The listing builds one solid part. Answer for the finished solid, in the listing's coordinates (mm). A direction names the side the tool comes from. Give positions to 0.01 mm unless a question says otherwise; leave off trailing zeros. Loops run counter-clockwise (first coordinate to the right, second up) from the corner with the lowest first, then second, coordinate; pieces in that order, holes last. Notation, with made-up numbers: M -39.5,83 L -21.5,83 A24 ccw -21.5,102 Z; hole C -26,-23.5 d9. An arc over 180 degrees is marked long. Return JSON: item names as keys, results as strings.
from build123d import *

# Parameters (mm, degrees)
SCHIZZO16_W                   = 10
SCHIZZO16_H                   = 180
SCHIZZO17_R                   = 20
ESTRUSIONE_ESTRUSIONE10_DEPTH = 12.75569081
SCHIZZO18_R                   = 8.5
ESTRUSIONE_ESTRUSIONE11_DEPTH = 32
SCHIZZO19_R                   = 6
ESTRUSIONE_ESTRUSIONE12_DEPTH = 44
SCHIZZO20_R                   = 5
ESTRUSIONE_ESTRUSIONE13_DEPTH = 10
SCHIZZO21_R                   = 4
ESTRUSIONE_ESTRUSIONE14_DEPTH = 12
SCHIZZO22_R                   = 20
ESTRUSIONE_ESTRUSIONE15_DEPTH = 11.80548778
SCHIZZO23_R                   = 7.4
ESTRUSIONE_ESTRUSIONE16_DEPTH = 61.8
SCHIZZO24_R                   = 5
ESTRUSIONE_ESTRUSIONE17_DEPTH = 10
RACCORDO1_R                   = 100


with BuildPart() as part:
    # Sweep1: sweep along a path in Schizzo15
    with BuildLine(Plane(origin=(0, 0, 0), x_dir=(1, 0, 0), z_dir=(0, 1, 0))) as sweep1_path:
        Line((-350, 35.20194684), (-190, 35.20194684))
        Line((-190, 35.20194684), (-80, 0))
        Line((-80, 0), (80, 0))
    # Schizzo16 → Sweep1 (sweep)
    with BuildSketch(Plane(origin=(0, 0, 0), x_dir=(0, 0, -1), z_dir=(1, 0, 0))):
        Rectangle(SCHIZZO16_W, SCHIZZO16_H)
    sweep(path=sweep1_path.line, transition=Transition.RIGHT)

    # Schizzo17 → Estrusione-Estrusione10 (add)
    with BuildSketch(Plane.XY.offset(5)):
        Circle(SCHIZZO17_R)
    extrude(amount=ESTRUSIONE_ESTRUSIONE10_DEPTH)

    # Schizzo18 → Estrusione-Estrusione11 (add)
    with BuildSketch(Plane.XY.offset(17.75569081)):
        Circle(SCHIZZO18_R)
    extrude(amount=ESTRUSIONE_ESTRUSIONE11_DEPTH)

    # Schizzo19 → Estrusione-Estrusione12 (add)
    with BuildSketch(Plane.XY.offset(49.75569081)):
        Circle(SCHIZZO19_R)
    extrude(amount=ESTRUSIONE_ESTRUSIONE12_DEPTH)

    # Schizzo20 → Estrusione-Estrusione13 (add)
    with BuildSketch(Plane.XY.offset(93.75569081)):
        Circle(SCHIZZO20_R)
    extrude(amount=ESTRUSIONE_ESTRUSIONE13_DEPTH)

    # Schizzo21 → Estrusione-Estrusione14 (add)
    with BuildSketch(Plane.XY.offset(103.75569081)):
        Circle(SCHIZZO21_R)
    extrude(amount=ESTRUSIONE_ESTRUSIONE14_DEPTH)

    # Schizzo22 → Estrusione-Estrusione15 (add)
    with BuildSketch(Plane.XY.offset(-30.20194684)):
        with Locations((-270, 0)):
            Circle(SCHIZZO22_R)
    extrude(amount=ESTRUSIONE_ESTRUSIONE15_DEPTH)

    # Schizzo23 → Estrusione-Estrusione16 (add)
    with BuildSketch(Plane.XY.offset(-18.39645906)):
        with Locations((-270, 0)):
            Circle(SCHIZZO23_R)
    extrude(amount=ESTRUSIONE_ESTRUSIONE16_DEPTH)

    # Schizzo24 → Estrusione-Estrusione17 (add)
    with BuildSketch(Plane.XY.offset(43.40354094)):
        with Locations((-270, 0)):
            Circle(SCHIZZO24_R)
    extrude(amount=ESTRUSIONE_ESTRUSIONE17_DEPTH)

    # Raccordo1
    raccordo1_edges = [part.edges().sort_by_distance(p)[0] for p in [
        (-80.78054705, 0, 5),
        (-190.78054705, 0, -30.20194684),
    ]]
    fillet(raccordo1_edges, radius=RACCORDO1_R)


solid = part.part
(1) Straight lines are drawn through the part: line 1 along Z through (x, y) = (-316, 12.5); line 2 along Z through (x, y) = (-59.5, -66.5). For each, find the intervals that lie inside material, in ascending order.
Values follow:
{"line 1": "-40.2 to -30.2", "line 2": "-5 to 5"}
(2) The part is cut by section C-C (z = 37). Determine the outline of the cut face in (x, y), and give its area (3 significant figures).
Values follow:
{"outline": "C -270,0 d14.8; C 0,0 d17", "area": "399 mm²"}
(3) Given pin 1 (10 mm diameter, centred on x = -123.5, y = -25, fed in from +Z); pin 2 (4.5 mm diameter, centred on x = -272, y = -3, fed in from +Z); pin 3 (1 mm diameter, centred on x = -150.5, y = 1, fed in from -Z), each flat-ended and moving along its own axis, determine where each tip first touches the part or whether it passes through.
Values follow:
{"pin 1": "z = -7.07", "pin 2": "z = 53.4", "pin 3": "z = -27.97"}
(4) The part is cut by section B-B (y = 64.5). Determine the outline of the cut face in (x, z).
Values follow:
{"outline": "M -350,-40.2 L -189.22,-40.2 L -79.22,-5 L 80,-5 L 80,5 L -65.17,5 A100 ccw -95.65,0.24 L -175.91,-25.44 A100 cw -206.39,-30.2 L -350,-30.2 Z"}
(5) The part is cut by section D-D (z = 85.5). Determine the outline of the cut face in (x, y).
Values follow:
{"outline": "C 0,0 d12"}
(6) The part is cut by section A-A (x = 0). Determine the outline of the cut face in (y, z), and give its area (3 significant figures).
Values follow:
{"outline": "M -90,-5 L 90,-5 L 90,5 L 20,5 L 20,17.76 L 8.5,17.76 L 8.5,49.76 L 6,49.76 L 6,93.76 L 5,93.76 L 5,103.76 L 4,103.76 L 4,115.76 L -4,115.76 L -4,103.76 L -5,103.76 L -5,93.76 L -6,93.76 L -6,49.76 L -8.5,49.76 L -8.5,17.76 L -20,17.76 L -20,5 L -90,5 Z", "area": "3,580 mm²"}
(7) Determine the mould class of faces 1 (the cylindrical face through (-251.525, -7.66, -24.382)), 2 (the flat face through (-4, 4, 93.756)), 3 (the flat face through (-135.22, 1.26, -12.42)), 4 (the flat face through (80, -1, 0)) for opening direction X: released by +X, released by -X, zero draft, split by the parting line, or undercut.
Values follow:
{"face 1": "undercut", "face 2": "zero draft", "face 3": "undercut", "face 4": "released by +X"}
(8) A tool of negligible diameter and unlimited length cuts with its end or side. For faces 5 (the cylindrical face through (-265.23, 1.5, 48.33)), 6 (the cylindrical face through (-191.18, -1.26, -29.04)), 7 (the flat face through (-134, 90, -18)), 8 (the flat face through (-350, -1, -35)), 9 (the flat face through (-270, 0, 53.404)), from which of +Z, -Z, +X, -X, +Y, -Y can it reach the whole face along a straight path? Write none if from no direction.
Values follow:
{"face 5": "+Z", "face 6": "+Z, +Y, -Y", "face 7": "+Z, -Z, +X, -X, +Y", "face 8": "+Z, -Z, -X, +Y, -Y", "face 9": "+Z, -X, +Y, -Y"}
